Check sheet for the modelled part. Datum: model origin and axes. Units: mm. A direction names the side the tool comes from. Round coordinates to 2 decimals unless told otherwise and drop trailing zeros. Write each loop counter-clockwise with the first axis right and the second up, starting at its lowest first coordinate (ties: lowest second). Pieces come first, ordered by that corner, then holes.
Item 1: Cross-section at D-D on z = 70.5. Enter the section's corners in (x, y), plus the area to 3 significant figures.
Item 2: Material ranges on line 1 (X direction, y = 6.5, z = 66); line 2 (Y direction, x = -93, z = 24); line 3 (Y direction, x = 110, z = 52), recorded low to high.
Item 3: Cross-section at B-B on z = 37. Enter the section's corners in (x, y), plus the area to 3 significant figures.
Item 4: Cross-section at A-A on x = 98.5. Enter the section's corners in (y, z).
Item 5: Cross-section at C-C on y = 0. Enter the section's corners in (x, z), plus the area to 3 significant figures.
Item 6: Release check for a two-part mould opening along Z. For faces 4 (the flat face through (-2, -15, 25)), 5 (the flat face through (110, 0, 45)), 6 (the flat face through (-140, 15, 60)) record: +Z half, -Z half, draft (parallel to the pull), parting line (faces both ways), or undercut.
Item 7: Tool access check on faces 1 (the flat face through (-2, 0, 10)), 2 (the flat face through (-2, 25, 37)), 3 (the flat face through (140, 0, 45)). Record the directions out of +Z, -Z, +X, -X, +Y, -Y that give a thin tool (end or side, any length) a straight path to the whole face; none if there is none.
Item 8: Go/stop test with flat-tipped pins: pin 1 Ø13 at (x, y) = (110, 0) entering from +Z; pin 2 Ø9 at (x, y) = (-141.5, 3.5) entering from +Z. Record where each tip stops, or that it passes through.
from build123d import *

# Parameters (mm, degrees)
CROQUIS1_W              = 330
CROQUIS1_H              = 50
SALIENTE_EXTRUIR1_DEPTH = 75
CROQUIS2_R              = 4
CROQUIS2_W              = 30
CROQUIS2_H              = 30
CORTAR_EXTRUIR1_DEPTH   = 30
CROQUIS3_W              = 30
CROQUIS3_H              = 30
CORTAR_EXTRUIR2_DEPTH   = 331


with BuildPart() as part:
    # Croquis1 → Saliente-Extruir1 (new body)
    with BuildSketch(Plane.XY):
        Rectangle(CROQUIS1_W, CROQUIS1_H)
    extrude(amount=SALIENTE_EXTRUIR1_DEPTH)

    # Croquis2 → Cortar-Extruir1 (cut)
    with BuildSketch(Plane.XY.offset(75)):
        with Locations((-110, 0)):
            Circle(CROQUIS2_R)
        with Locations((110, 0)):
            Circle(CROQUIS2_R)
        with Locations((-140, 0)):
            Rectangle(CROQUIS2_W, CROQUIS2_H)
        with Locations((140, 0)):
            Rectangle(CROQUIS2_W, CROQUIS2_H)
    extrude(amount=-CORTAR_EXTRUIR1_DEPTH, mode=Mode.SUBTRACT)

    # Croquis3 → Cortar-Extruir2 (cut, through all)
    with BuildSketch(Plane.ZY.offset(165)):
        with Locations((25, 0)):
            Rectangle(CROQUIS3_W, CROQUIS3_H)
    extrude(amount=-CORTAR_EXTRUIR2_DEPTH, mode=Mode.SUBTRACT)


solid = part.part
Response values:
1. outline: (-165, -25) - (165, -25) - (165, 25) - (-165, 25) - close; hole (-155, -15) - (-125, -15) - (-125, 15) - (-155, 15) - close; hole circle Ø8 at (-110, 0); hole circle Ø8 at (110, 0); hole (125, -15) - (155, -15) - (155, 15) - (125, 15) - close
1. area: 14,600 mm2
2. line 1: x = -165 to -155, -125 to 125, 155 to 165
2. line 2: y = -25 to -15, 15 to 25
2. line 3: y = -25 to -4, 4 to 25
3. outline: (-165, -25) - (165, -25) - (165, -15) - (-165, -15) - close; (-165, 15) - (165, 15) - (165, 25) - (-165, 25) - close
3. area: 6,600 mm2
4. outline: (-25, 0) - (25, 0) - (25, 75) - (-25, 75) - close; hole (-15, 10) - (15, 10) - (15, 40) - (-15, 40) - close
5. outline: (-165, 0) - (165, 0) - (165, 10) - (-165, 10) - close; (-165, 40) - (165, 40) - (165, 75) - (155, 75) - (155, 45) - (125, 45) - (125, 75) - (114, 75) - (114, 45) - (106, 45) - (106, 75) - (-106, 75) - (-106, 45) - (-114, 45) - (-114, 75) - (-125, 75) - (-125, 45) - (-155, 45) - (-155, 75) - (-165, 75) - close
5. area: 12,600 mm2
6. face 4: undercut
6. face 5: +Z half
6. face 6: draft
7. face 1: +X, -X
7. face 2: +Z, -Z, +X, -X, +Y
7. face 3: +Z
8. pin 1: stops at z = 75
8. pin 2: stops at z = 45
